Job drawing, mm, ordinate dimensions from the low corner. One solid piece. A direction names the side the tool comes from. Coordinates: 2 decimals unless noted, no trailing zeros. Order: outer loops, then holes, each group sorted by start corner. A loop starts at its lowest first (then second) coordinate and runs counter-clockwise, first axis right, second up. Notation, with made-up numbers: (8, 26) - (24, 26) arc R8 ccw to (24, 39) - close; hole circle Ø5 at (88, 32). An arc over 180 degrees is marked (long way). Return JSON: item names as keys, results as strings.
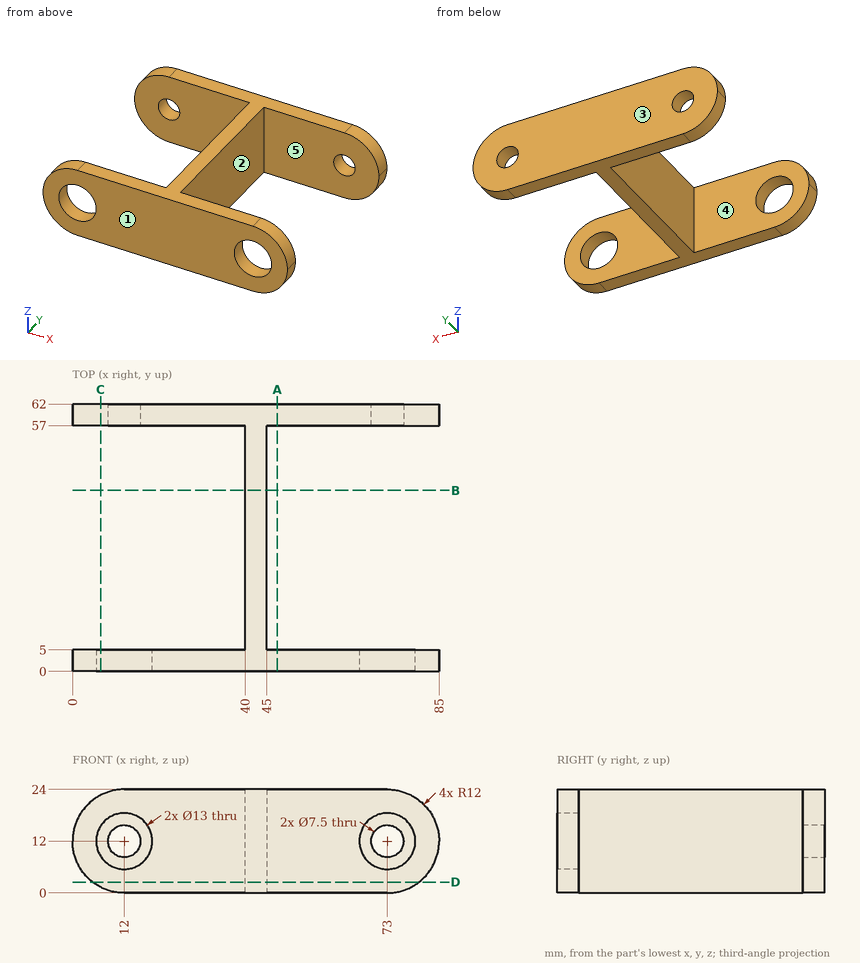
1. Cut at A-A on x = 47.5. Give the cut face in (y, z).
Check values:
{"outline": "(0, 0) - (5, 0) - (5, 24) - (0, 24) - close; (57, 0) - (62, 0) - (62, 24) - (57, 24) - close"}
2. Cut at D-D on z = 2.5. Give the cut face in (x, y).
Check values:
{"outline": "(4.67, 0) - (80.33, 0) - (80.33, 5) - (45, 5) - (45, 57) - (80.33, 57) - (80.33, 62) - (4.67, 62) - (4.67, 57) - (40, 57) - (40, 5) - (4.67, 5) - close"}
3. Cut at B-B on y = 42. Give the cut face in (x, z), plus the area to 3 significant figures.
Check values:
{"outline": "(40, 0) - (45, 0) - (45, 24) - (40, 24) - close", "area": "120 mm²"}
4. Cut at C-C on x = 6.5. Give the cut face in (y, z), plus the area to 3 significant figures.
Check values:
{"outline": "(0, 1.33) - (5, 1.33) - (5, 8.54) - (0, 8.54) - close; (0, 15.46) - (5, 15.46) - (5, 22.67) - (0, 22.67) - close; (57, 1.33) - (62, 1.33) - (62, 22.67) - (57, 22.67) - close", "area": "179 mm²"}
5. Drop flat-ended pins along their axis: pin 1 (1 mm diameter, centred on y = 38.5, z = 5.5, fed in from -X); pin 2 (8.5 mm diameter, centred on x = 73, z = 12, fed in from -Y); pin 3 (8 mm diameter, centred on y = 24.5, z = 3.5, fed in from +X). Give the stop position or say it passes through.
Check values:
{"pin 1": "x = 40", "pin 2": "y = 57", "pin 3": "x = 45"}
6. Mould opens along Y. For the marked faces 1, 2 and 3 say: pulls with the +Y half, pulls with the -Y half, needs draft (parallel to the pull), parting line crosses it, or undercut.
Check values:
{"face 1": "pulls with the -Y half", "face 2": "undercut", "face 3": "pulls with the +Y half"}
7. Probe L1, parallel to X at y = 60.15, z = 12; L2, parallel to Y at x = 77, z = 22.75; L3, parallel to Z at x = 12, y = 58.5. List the from-to ranges inside material, lowest first.
Check values:
{"L1": "0 to 8.25, 15.75 to 69.25, 76.75 to 85", "L2": "0 to 5, 57 to 62", "L3": "0 to 8.25, 15.75 to 24"}
8. Tool access for the marked faces 4 and 5: list every direction of +Z, -Z, +X, -X, +Y, -Y with a clear straight run to the whole face (end or side of a thin tool).
Check values:
{"face 4": "+Z, -Z, -X", "face 5": "+Z, -Z, +X"}
